Can you work these out from the model? Positions are in its coordinate system, mm. A direction names the side the tool comes from. Give positions to 0.01 mm unless a question says otherwise; leave off trailing zeros. Write each loop counter-clockwise with the first axis right and the second up, starting at its lowest first coordinate (ties: lowest second). Pieces come first, ordered by that corner, then holes.
Autodesk Fusion 360 part; units mm, degrees
sketch "Sketch1" plane through (0, 0, 0) normal (0, 0, 1) x (1, 0, 0)
  circle A0 centre (0, 0) radius 65
  dimension "d1" = 130
extrude "Extrude1" add sketch "Sketch1" along normal blind 12.7
hole "Hole1" at (0.1314, 0.2629, 12.7) direction (0, 0, -1) diameter 76.2 depth 5 tip angle 180
hole "Hole2" at (-28.552, 0.2545, 7.7) direction (0, 0, -1) diameter 7 depth 7.7 tip angle 180
hole "Hole3" at (-0.3573, -30.3398, 7.7) direction (0, 0, -1) diameter 7 depth 7.7 tip angle 180
hole "Hole4" at (-0.4431, 30.9664, 7.7) direction (0, 0, -1) diameter 7 depth 7.7 tip angle 180
hole "Hole5" at (30.8296, -0.3123, 7.7) direction (0, 0, -1) diameter 7 depth 7.7 tip angle 180
sketch "Sketch2" plane through (0, 0, 0) normal (0, 0, 1) x (1, 0, 0)
sketch "Sketch3" plane through (0, 0, 12.7) normal (0, 0, 1) x (-1, 0, 0)
  circle A0 centre (-0.1314, -0.2629) radius 38.1
  circle A1 centre (0, 0) radius 65
(1) Will these pins go through, and if not, where does the flat tip stop? P1, Ø2, axis at x = 26, z = 10, coming from the +Y side; P2, Ø9, axis at x = 30.83, y = -0.31, coming from the -Z side; P3, Ø1, axis at y = -38.5, z = 3, coming from the +X side; P4, Ø2, axis at x = -35.5, z = 5, coming from the -Y side.
Returned:
P1: stops at y = 60
P2: stops at z = 0
P3: stops at x = 52.74
P4: stops at y = -55.09
(2) For faces 1 (the face through (-11.31, -36.08, 10.16)), 2 (the face through (27.36, 0.14, 3.8)), which set-ups out of +Z, -Z, +X, -X, +Y, -Y let a thin tool reach every point of the face, with its end or its side?
Returned:
face 1: +Z
face 2: +Z, -Z
(3) If we mould it in two halves opening along X, with no side actions, what happens to faces 3 (the face through (62, -19.52, 6.26)), 4 (the face through (0, 1, 7.7)), 5 (the face through (-1, 1, 0))? For each: +X half, -X half, draft (parallel to the pull), parting line (faces both ways), or undercut.
Returned:
face 3: parting line
face 4: undercut
face 5: draft
(4) Imagine slicing it at B-B, the plane z = 6. Write out the boundary of the cut face in (x, y), plus the area to 3 significant figures.
Returned:
outline: circle Ø130 at (0, 0); hole circle Ø7 at (-28.55, 0.25); hole circle Ø7 at (-0.44, 30.97); hole circle Ø7 at (-0.36, -30.34); hole circle Ø7 at (30.83, -0.31)
area: 13,100 mm2
(5) Imagine slicing it at D-D, the plane y = -23.5. Write out the boundary of the cut face in (x, z), plus the area to 3 significant figures.
Returned:
outline: (-60.6, 0) - (60.6, 0) - (60.6, 12.7) - (29.91, 12.7) - (29.91, 7.7) - (-29.65, 7.7) - (-29.65, 12.7) - (-60.6, 12.7) - close
area: 1,240 mm2
(6) Imagine slicing it at A-A, the plane y = 0. Write out the boundary of the cut face in (x, z), plus the area to 3 significant figures.
Returned:
outline: (-65, 0) - (-32.04, 0) - (-32.04, 7.7) - (-37.97, 7.7) - (-37.97, 12.7) - (-65, 12.7) - close; (-25.06, 0) - (27.34, 0) - (27.34, 7.7) - (-25.06, 7.7) - close; (34.32, 0) - (65, 0) - (65, 12.7) - (38.23, 12.7) - (38.23, 7.7) - (34.32, 7.7) - close
area: 1,160 mm2
(7) Imagine slicing it at C-C, the plane x = -14.5. Write out the boundary of the cut face in (y, z), plus the area to 3 significant figures.
Returned:
outline: (-63.36, 0) - (63.36, 0) - (63.36, 12.7) - (35.44, 12.7) - (35.44, 7.7) - (-34.92, 7.7) - (-34.92, 12.7) - (-63.36, 12.7) - close
area: 1,260 mm2
(8) If I drill on L1, parallel to X at y = 2.5, z = 3.5; L2, parallel to X at y = 29, z = 11.5; L3, parallel to Y at x = 31.5, z = 10.5, over which ranges is the centre line in solid material (lowest first)?
Returned:
L1: x = -64.95 to -31.24, -25.87 to 28.75, 32.91 to 64.95
L2: x = -58.17 to -24.88, 25.15 to 58.17
L3: y = -56.86 to -21.36, 21.89 to 56.86
